The listing builds one solid part. Answer for the finished solid, in the listing's coordinates (mm). Face numbers are marked on the shaded views. A direction names the side the tool comes from. Give positions to 0.01 mm unless a question says otherwise; leave off trailing zeros. Write each loop counter-clockwise with the first axis right and the second up, starting at its lowest first coordinate (ties: lowest second). Pieces come first, ordered by that corner, then holes. Notation, with made-up numbers: (7, 13.5) - (16, 13.5) arc R16 cw to (16, 30.5) - close; hole circle Ø10 at (70.25, -28). An arc over 180 degrees is marked (long way). One line per item, written item: value. Start each with the question number.
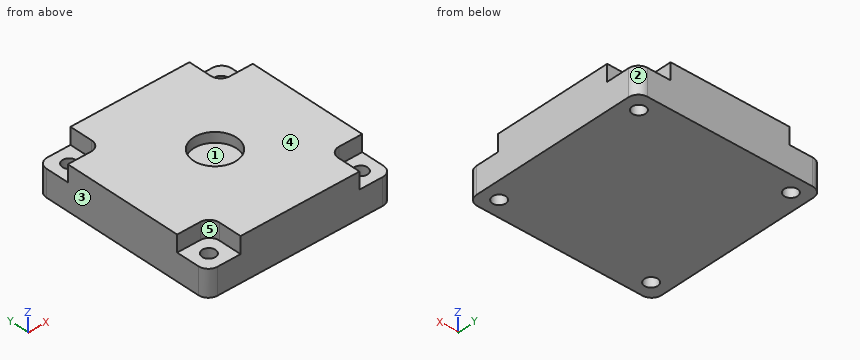
Autodesk Inventor part; units mm, degrees
ref_plane "YZ Plane" through (0, 0, 0) normal (1, 0, 0) x (0, 1, 0)
ref_plane "XZ Plane" through (0, 0, 0) normal (0, 1, 0) x (-1, 0, 0)
ref_plane "XY Plane" through (0, 0, 0) normal (0, 0, 1) x (1, 0, 0)
sketch "Sketch1" plane through (0, 0, 0) normal (0, 0, 1) x (1, 0, 0)
  line L0 (0, 0) -> (28, 0)
  line L1 (28, 0) -> (28, 28)
  line L2 (28, 28) -> (0, 28)
  line L3 (0, 28) -> (0, 0)
  dimension "d0" = 28
  dimension "d1" = 28
extrude "Extrusion1" add sketch "Sketch1" along normal blind 6.5
sketch "Sketch6" plane through (0, 0, 6.5) normal (0, 0, 1) x (1, 0, 0)
  line L0 (0, 0) -> (5, 0)
  line L1 (5, 0) -> (5, 5)
  line L2 (5, 5) -> (0, 5)
  line L3 (0, 5) -> (0, 0)
  line L4 (23, 5) -> (28, 5)
  line L5 (28, 5) -> (28, 0)
  line L6 (28, 0) -> (23, 0)
  line L7 (23, 0) -> (23, 5)
  line L8 (0, 28) -> (5, 28)
  line L9 (5, 28) -> (5, 23)
  line L10 (5, 23) -> (0, 23)
  line L11 (0, 23) -> (0, 28)
  line L12 (28, 28) -> (23, 28)
  line L13 (23, 28) -> (23, 23)
  line L14 (23, 23) -> (28, 23)
  line L15 (28, 23) -> (28, 28)
  dimension "d28" = 5
  dimension "d29" = 5
  dimension "d30" = 5
  dimension "d31" = 5
  dimension "d32" = 5
extrude "Extrusion4" cut sketch "Sketch6" against normal blind 2.5
fillet "Fillet2" radius 1.5 8 edges at (0, 0, 2) (5, 5, 5.25) (0, 28, 2) (5, 23, 5.25) (23, 23, 5.25) (28, 28, 2) (23, 5, 5.25) (28, 0, 2)
sketch "Sketch7" plane through (0, 0, 4) normal (0, 0, 1) x (1, 0, 0)
  line L0 (0, 23) -> (0, 26.5)
  line L1 (1.5, 28) -> (5, 28)
  line L2 (5, 0) -> (1.5, 0)
  line L3 (28, 23) -> (28, 5)
  line L4 (0, 1.5) -> (0, 5)
  line L5 (5, 28) -> (23, 28)
  line L6 (23, 0) -> (5, 0)
  point P0 (2.5, 25.5)
  point P1 (2.5, 2.5)
  point P2 (25.5, 25.5)
  point P3 (25.5, 2.5)
  dimension "d36" = 2.5
  dimension "d37" = 2.5
  dimension "d38" = 2.5
  dimension "d39" = 2.5
  dimension "d52" = 2.5
  dimension "d53" = 2.5
  dimension "d54" = 2.5
  dimension "d55" = 2.5
hole "Hole2" at (2.5, 25.5, 4) at (2.5, 2.5, 4) at (25.5, 25.5, 4) at (25.5, 2.5, 4) direction (0, 0, -1) diameter 2.013 end through all
sketch "Sketch8" plane through (0, 0, 6.5) normal (0, 0, 1) x (1, 0, 0)
  line L0 (5, 28) -> (23, 28)
  line L1 (0, 5) -> (0, 23)
  circle A0 centre (14, 14) radius 3.25
  dimension "d47" = 6.5
  dimension "d48" = 14
  dimension "d49" = 14
extrude "Extrusion5" cut sketch "Sketch8" against normal blind 1.5
properties part number "stepper_bottom_28"
Item 1: Find section A-A on y = 25.5. Determine the outline of the cut face in (x, z).
Item 2: Find section C-C on z = 5.75. Determine the outline of the cut face in (x, y), plus the area to 3 significant figures.
Item 3: Each of these flat-tipped pins is pushed along its axis until it touches: pin 1 Ø1.5 at (x, y) = (1.5, 2) entering from +Z; pin 2 Ø3 at (y, z) = (26, 5) entering from +X; pin 3 Ø1.2 at (x, z) = (1, 5) entering from +Y; pin 4 Ø6 at (x, y) = (14, 14) entering from +Z. Where does it stop, or does it pass through?
Item 4: Find section B-B on x = 14. Determine the outline of the cut face in (y, z), plus the area to 3 significant figures.
Item 5: Straight lines are drawn through the part: line 1 along Y through (x, z) = (2.5, 2.9); line 2 along Y through (x, z) = (14, 5.35). For each, find the intervals that lie inside material, in ascending order.
Item 6: Find section D-D on x = 25. Determine the outline of the cut face in (y, z).
Item 7: For the marked faces 4 and 5, determine the directions among +Z, -Z, +X, -X, +Y, -Y from which every point of the face is accessible in a straight line to the end or side of a thin tool.
Item 8: The mould has two halves that part along X. Classify the marked faces 1, 2 and 3: +X half, -X half, draft (parallel to the pull), parting line (faces both ways), or undercut.
Values:
1. outline: (0, 0) - (1.49, 0) - (1.49, 4) - (0, 4) - close; (3.51, 0) - (24.49, 0) - (24.49, 4) - (23, 4) - (23, 6.5) - (5, 6.5) - (5, 4) - (3.51, 4) - close; (26.51, 0) - (28, 0) - (28, 4) - (26.51, 4) - close
2. outline: (0, 5) - (3.5, 5) arc R1.5 cw to (5, 3.5) - (5, 0) - (23, 0) - (23, 3.5) arc R1.5 cw to (24.5, 5) - (28, 5) - (28, 23) - (24.5, 23) arc R1.5 cw to (23, 24.5) - (23, 28) - (5, 28) - (5, 24.5) arc R1.5 cw to (3.5, 23) - (0, 23) - close; hole circle Ø6.5 at (14, 14)
2. area: 653 mm^2
3. pin 1: z = 4
3. pin 2: x = 28
3. pin 3: y = 23
3. pin 4: z = 5
4. outline: (0, 0) - (28, 0) - (28, 6.5) - (17.25, 6.5) - (17.25, 5) - (10.75, 5) - (10.75, 6.5) - (0, 6.5) - close
4. area: 172 mm^2
5. line 1: 0 to 1.49, 3.51 to 24.49, 26.51 to 28
5. line 2: 0 to 10.75, 17.25 to 28
6. outline: (0, 0) - (1.63, 0) - (1.63, 4) - (0, 4) - close; (3.37, 0) - (24.63, 0) - (24.63, 4) - (23, 4) - (23, 6.5) - (5, 6.5) - (5, 4) - (3.37, 4) - close; (26.37, 0) - (28, 0) - (28, 4) - (26.37, 4) - close
7. face 4: +Z, +X, -X, +Y, -Y
7. face 5: +Z, -X, -Y
8. face 1: undercut
8. face 2: +X half
8. face 3: -X half
